from build123d import *

# Parameters (mm, degrees)
F0_W      = 30
F0_H      = 26
F1_DEPTH  = 15
F3_SIZE2  = 2
F3_SIZE   = 1.5
F5_DEPTH  = 30.001
F6_SIZE   = 4
F2_W      = 21.5
F2_H      = 7
F7_DEPTH  = 12
F8_W      = 11
F8_H      = 7
F9_DEPTH  = 4
F10_R     = 5
F11_R     = 5
F12_W     = 30
F12_H     = 5
F13_DEPTH = 15.001
F15_D     = 4.4
F16_W     = 27
F16_H     = 10
F16_W_2   = 15
F16_H_2   = 19
F17_DEPTH = 4


with BuildPart() as f1:
    # F0 (on Top) → F1 (new body)
    with BuildSketch(Plane.XY):
        Rectangle(F0_W, F0_H)
    extrude(amount=F1_DEPTH)

    # F3
    f3_edges = [f1.edges().sort_by_distance(p)[0] for p in [
        (-15, -13, 7.5),
        (15, -13, 7.5),
    ]]
    f3_side = f1.faces().sort_by_distance((0, -13, 7.5))[0]
    chamfer(f3_edges, length=F3_SIZE, length2=F3_SIZE2, reference=f3_side)

    # F4 (on face) → F5 (cut, through all)
    with BuildSketch(Plane(origin=(-15, 0, 0), x_dir=(0, -1, 0), z_dir=(-1, 0, 0))):
        Polygon((-13, 12), (-13, 0), (-8, 0), (-8, 4), (-3, 4), (-3, 12), align=None)
    extrude(amount=-F5_DEPTH, mode=Mode.SUBTRACT)

    # F6
    f6_edges = [f1.edges().sort_by_distance(p)[0] for p in [
        (-15, 3, 8),
        (15, 3, 8),
    ]]
    chamfer(f6_edges, length=F6_SIZE)

    # F2 (on face) → F7 (cut)
    with BuildSketch(Plane.XZ.offset(13)):
        with Locations((0, 7.5)):
            Rectangle(F2_W, F2_H)
    extrude(amount=-F7_DEPTH, mode=Mode.SUBTRACT)

    # F8 (on face) → F9 (cut)
    with BuildSketch(Plane(origin=(0, 3, 0), x_dir=(-1, 0, 0), z_dir=(0, 1, 0))):
        with Locations((0, 8)):
            Rectangle(F8_W, F8_H)
    extrude(amount=-F9_DEPTH, mode=Mode.SUBTRACT)

    # F10
    f10_edges = [f1.edges().sort_by_distance(p)[0] for p in [
        (-10.75, -1, 7.5),
    ]]
    fillet(f10_edges, radius=F10_R)

    # F11
    f11_edges = [f1.edges().sort_by_distance(p)[0] for p in [
        (10.75, -1, 7.5),
    ]]
    fillet(f11_edges, radius=F11_R)

    # F12 (on face) → F13 (cut, through all)
    with BuildSketch(Plane.XY.offset(15)):
        with Locations((0, 10.5)):
            Rectangle(F12_W, F12_H)
    extrude(amount=-F13_DEPTH, mode=Mode.SUBTRACT)

    # F15 (through all)
    with Locations(Plane.XY.offset(15)):
        with Locations((0, -9.5)):
            Hole(F15_D / 2)

    # F16 (on face) → F17 (join)
    with BuildSketch(Plane(origin=(0, 0, 0), x_dir=(1, 0, 0), z_dir=(0, 0, -1))):
        with Locations((0, 18)):
            Rectangle(F16_W, F16_H)
        with Locations((22.5, 1.5)):
            Rectangle(F16_W_2, F16_H_2)
        with BuildLine():
            Line((19.75, -1.5), (19.75, 4.5))
            ThreePointArc((19.75, 4.5), (22.5, 7.25), (25.25, 4.5))
            Line((25.25, 4.5), (25.25, -1.5))
            ThreePointArc((25.25, -1.5), (22.5, -4.25), (19.75, -1.5))
        make_face(mode=Mode.SUBTRACT)
        with Locations((-22.5, 1.5)):
            Rectangle(F16_W_2, F16_H_2)
        with BuildLine():
            ThreePointArc((-25.25, 4.5), (-22.5, 7.25), (-19.75, 4.5))
            Line((-19.75, 4.5), (-19.75, -1.5))
            ThreePointArc((-19.75, -1.5), (-22.5, -4.25), (-25.25, -1.5))
            Line((-25.25, -1.5), (-25.25, 4.5))
        make_face(mode=Mode.SUBTRACT)
    extrude(amount=-F17_DEPTH)


solid = f1.part
Could you check a few things on this model? Use its own coordinates, in mm. A direction names the side the tool comes from. Coordinates: 2 decimals unless noted, no trailing zeros. Write each loop counter-clockwise with the first axis right and the second up, starting at its lowest first coordinate (ties: lowest second). Pieces come first, ordered by that corner, then holes. Notation, with made-up numbers: M -7.5,-9 L 40.5,-9 A27 cw 40.5,11 Z; hole C 8,18 d9. An arc over 180 degrees is marked long. One line per question, with ' | ' between items.
1) Imagine slicing it at C-C, the plane z = 10.25. Write out the boundary of the cut face in (x, y).
Checks:
outline: M -15,-11 L -13.5,-13 L -10.75,-13 L -10.75,-6 A5 cw -5.75,-1 L -5.5,-1 L -5.5,3 L -11,3 L -15,-1 Z; M 5.5,-1 L 5.75,-1 A5 cw 10.75,-6 L 10.75,-13 L 13.5,-13 L 15,-11 L 15,-1 L 11,3 L 5.5,3 Z
2) I need wall thicknesses on probe 1 along Y at (x, z) = (0, 12.75); probe 2 along Z at (x, y) = (3.5, -4.5); probe 3 along Y at (x, z) = (0, 1.15). Which ranges of each line are inside material? Lowest first, please. Write a range as [from, to].
Checks:
probe 1: [-13, -11.7], [-7.3, 8] | probe 2: [0, 4], [11, 15] | probe 3: [-23, -11.7], [-7.3, 8]
3) Imagine slicing it at D-D, the plane z = 2.5. Write out the boundary of the cut face in (x, y).
Checks:
outline: M -30,-11 L -15,-11 L -13.5,-13 L -13.5,-23 L 13.5,-23 L 13.5,-13 L 15,-11 L 30,-11 L 30,8 L -30,8 Z; hole M -25.25,-4.5 A2.75 ccw -19.75,-4.5 L -19.75,1.5 A2.75 ccw -25.25,1.5 Z; hole C 0,-9.5 d4.4; hole M 19.75,-4.5 A2.75 ccw 25.25,-4.5 L 25.25,1.5 A2.75 ccw 19.75,1.5 Z
4) For pin 1 Ø9 at (y, z) = (-1, 8) entering from +X; pin 2 Ø1.2 at (x, z) = (-25.5, 1.5) entering from -Y; pin 3 Ø4.5 at (y, z) = (2, 8) entering from -X; pin 4 Ø3 at (y, z) = (0.5, 12.5) entering from +X, each with a flat end and sliding along its axis, tell me the tip position at first contact or that it passes through.
Checks:
pin 1: x = 30 | pin 2: y = -11 | pin 3: x = -14.25 | pin 4: x = 15
5) If we mould it in two halves opening along Z, with no side actions, what happens to faces 1 (the face through (0, -12, 4)), 2 (the face through (0, -23, 2)), 3 (the face through (0, -4, 0))? For each: released by +Z, released by -Z, zero draft, split by the parting line, or undercut.
Checks:
face 1: undercut | face 2: zero draft | face 3: released by -Z
6) Imagine slicing it at A-A, the plane x = 0. Write out the boundary of the cut face in (y, z).
Checks:
outline: M -23,0 L -11.7,0 L -11.7,4 L -23,4 Z; M -13,11 L -11.7,11 L -11.7,15 L -13,15 Z; M -7.3,0 L 8,0 L 8,4 L 3,4 L 3,4.5 L -1,4.5 L -1,4 L -7.3,4 Z; M -7.3,11 L -1,11 L -1,11.5 L 3,11.5 L 3,12 L 8,12 L 8,15 L -7.3,15 Z
7) Imagine slicing it at B-B, the plane y = -9.5. Write out the boundary of the cut face in (x, z), and give its area (3 significant figures).
Checks:
outline: M -30,0 L -2.2,0 L -2.2,4 L -10.75,4 L -10.75,11 L -2.2,11 L -2.2,15 L -15,15 L -15,4 L -30,4 Z; M 2.2,0 L 30,0 L 30,4 L 15,4 L 15,15 L 2.2,15 L 2.2,11 L 10.75,11 L 10.75,4 L 2.2,4 Z | area: 384 mm²
8) For faces 4 (the face through (-13, 1, 8)), 5 (the face through (0, 1, 4.5)), 6 (the face through (13.5, -18, 2)), which set-ups out of +Z, -Z, +X, -X, +Y, -Y let a thin tool reach every point of the face, with its end or its side?
Checks:
face 4: -X, +Y | face 5: +Y, -Y | face 6: +Z, -Z, +X, -Y
